For this review, take the finished solid that the model builds, in its own axes (mm). Coordinates: 2 decimals unless noted, no trailing zeros. Loops run counter-clockwise (first coordinate to the right, second up) from the corner with the lowest first, then second, coordinate; pieces in that order, holes last. Notation, with made-up numbers: (22.25, -37) - (51.25, -37) arc R24 ccw to (51.25, -1) - close; hole circle Ø2 at (44, 62). An arc over 180 degrees is marked (long way). Answer as a JSON object with one key per item and string values. Group by question number.
Item 1: We need section B-B (z = 32). Give the boundary of the cut face in (x, y).
Item 2: We need section D-D (x = 19). Give the boundary of the cut face in (y, z).
Item 3: Clearance check with flat-ended pins moving along their axes: pin 1 (1 mm diameter, centred on y = 2.5, z = 30, fed in from +X); pin 2 (1.5 mm diameter, centred on x = -10, y = 1.5, fed in from -Z). State where each tip first meets the part, or that it passes through.
Item 4: We need section A-A (x = -18.5). Give the boundary of the cut face in (y, z).
Item 5: To check wall thickness, follow line 1 (X direction, y = 4.15, z = 15.5); line 2 (Z direction, x = -22.5, y = 0.85); line 3 (X direction, y = 1.05, z = -12). State the ranges of each line that lie inside material, in increasing order.
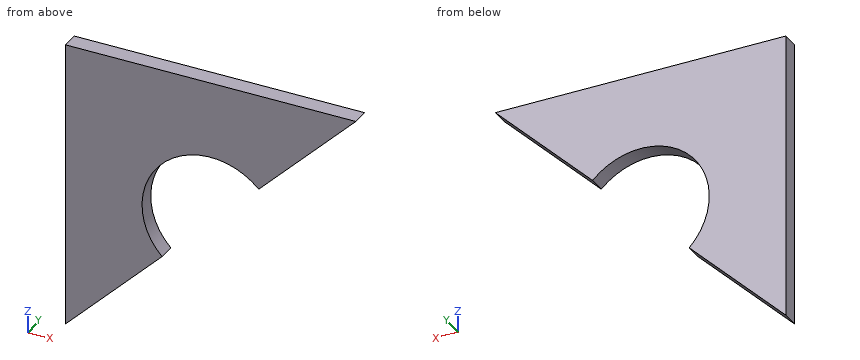
from build123d import *

# Parameters (mm, degrees)
BOSS_EXTRU_1_DEPTH = 5


with BuildPart() as part:
    # Esquisse1 → Boss.-Extru.1 (new body)
    with BuildSketch(Plane(origin=(0, 0, 0), x_dir=(1, 0, 0), z_dir=(0, 1, 0))):
        with BuildLine():
            Line((-14.220317816, 14.220317816), (-42.5, 42.5))
            Line((-42.5, 42.5), (-42.5, -42.5))
            Line((-42.5, -42.5), (42.5, -42.5))
            Line((42.5, -42.5), (14.063953431, -14.063953431))
            ThreePointArc((14.063953431, -14.063953431), (-14.220317816, -14.063953431), (-14.220317816, 14.220317816))
        make_face()
    extrude(amount=BOSS_EXTRU_1_DEPTH)


solid = part.part
Check sheet entries:
{
 "1": {"outline": "(-42.5, 0) - (32, 0) - (32, 5) - (-42.5, 5) - close"},
 "2": {"outline": "(0, 19) - (5, 19) - (5, 42.5) - (0, 42.5) - close"},
 "3": {"pin 1": "stops at x = 30.5", "pin 2": "stops at z = 16.84"},
 "4": {"outline": "(0, -18.5) - (5, -18.5) - (5, -7.87) - (0, -7.87) - close; (0, 7.71) - (5, 7.71) - (5, 42.5) - (0, 42.5) - close"},
 "5": {"line 1": "x = -42.5 to -12.62, 12.46 to 15.5", "line 2": "z = -22.5 to 42.5", "line 3": "x = -42.5 to -16.14"}
}
